CAD build for the part. Positions are in the model's coordinates, mm. A direction names the side the tool comes from. Coordinates: 2 decimals unless noted, no trailing zeros. Write each loop counter-clockwise with the first axis right and the second up, starting at its lowest first coordinate (ties: lowest second). Pieces come first, ordered by that corner, then holes. Notation, with made-up numbers: (60, 61) - (85, 61) arc R21 ccw to (85, 88) - close; hole circle Ø8 at (22.5, 62). An arc over 180 degrees is marked (long way). Answer in a Markdown table with one row per item. Add a question column.
Q1. Two-plate mould, pull along X, no slides. Class faces 5 (the flat face through (2, 6.35, 2)), 6 (the flat face through (47.997, 20, 2)): +X half, -X half, draft (parallel to the pull), parting line (faces both ways), or undercut.
Q2. Pin check, flat tips, straight feed: pin 1 (0.9 mm diameter, centred on y = 9, z = 2, fed in from -X) (3 decimals); pin 2 (1.6 mm diameter, centred on x = 11.5, z = 2, fed in from -Y) (3 decimals). Stop position of each tip, or through.
Q3. Band-saw the part on C-C (y = 5). State how many separate pieces and enclosed holes the cut face has, and give its area (3 significant figures).
Q4. Band-saw the part on B-B (x = 5). List the corners of the cut face in (y, z) (3 decimals), and give its area (3 significant figures).
Q5. 3-axis set-ups, long thin cutter, end or side, ignore diameter. For faces 1 (the flat face through (10, 25.4, 2)), 2 (the flat face through (2, 19.05, 2)), 3 (the flat face through (9.525, 9, 2)), 4 (the flat face through (15.875, 2, 2)): which of +Z, -Z, +X, -X, +Y, -Y reach the whole face in a straight line?
Q6. Drill centre lines: line 1 along Y through (x, z) = (4.5, 0.8) (3 decimals); line 2 along Y through (x, z) = (9, 1.95) (3 decimals). Where is each one in solid material? Low to high. Write a range as from..to.
Q7. Band-saw the part on A-A (x = 11). List the corners of the cut face in (y, z) (1 decimal).
```python
from build123d import *

# Parameters (mm, degrees)
BOSS_EXTRUDE2_DEPTH = 3.175


with BuildPart() as part:
    # Sketch1 → Boss-Extrude2 (new body)
    with BuildSketch(Plane.XY):
        Polygon((0, 6.35), (0, 0), (6.35, 0), (6.35, 3.175), (15.875, 3.175), (15.875, 0), (19.05, 0), (19.549044577, 11.43), (20.048089155, 0), (21.082, 0), (21.581044577, 11.43), (22.080089155, 0), (23.114, 0), (23.613044577, 11.43), (24.112089155, 0), (25.146, 0), (25.645044577, 11.43), (26.144089155, 0), (27.178, 0), (27.677044577, 11.43), (28.176089155, 0), (29.21, 0), (29.709044577, 11.43), (30.208089155, 0), (31.242, 0), (31.741044577, 11.43), (32.240089155, 0), (33.274, 0), (33.773044577, 11.43), (34.272089155, 0), (35.306, 0), (35.805044577, 11.43), (36.304089155, 0), (37.338, 0), (37.837044577, 11.43), (38.336089155, 0), (39.37, 0), (39.869044577, 11.43), (40.368089155, 0), (41.402, 0), (41.901044577, 11.43), (42.400089155, 0), (43.434, 0), (43.933044577, 11.43), (44.432089155, 0), (45.466, 0), (45.965044577, 11.43), (46.464089155, 0), (47.498, 0), (47.997044577, 11.43), (47.997044577, 0), (50.8, 0), (50.8, 25.4), (47.997044577, 25.4), (47.997044577, 13.97), (47.498, 25.4), (46.464089155, 25.4), (45.965044577, 13.97), (45.466, 25.4), (44.432089155, 25.4), (43.933044577, 13.97), (43.434, 25.4), (42.400089155, 25.4), (41.901044577, 13.97), (41.402, 25.4), (40.368089155, 25.4), (39.869044577, 13.97), (39.37, 25.4), (38.336089155, 25.4), (37.837044577, 13.97), (37.338, 25.4), (36.304089155, 25.4), (35.805044577, 13.97), (35.306, 25.4), (34.272089155, 25.4), (33.773044577, 13.97), (33.274, 25.4), (32.240089155, 25.4), (31.741044577, 13.97), (31.242, 25.4), (30.208089155, 25.4), (29.709044577, 13.97), (29.21, 25.4), (28.176089155, 25.4), (27.677044577, 13.97), (27.178, 25.4), (26.144089155, 25.4), (25.645044577, 13.97), (25.146, 25.4), (24.112089155, 25.4), (23.613044577, 13.97), (23.114, 25.4), (22.080089155, 25.4), (21.581044577, 13.97), (21.082, 25.4), (20.048089155, 25.4), (19.549044577, 13.97), (19.05, 25.4), (0, 25.4), (0, 19.05), (3.175, 19.05), (3.175, 14.605), (9.525, 14.605), (9.525, 17.4625), (12.7, 17.4625), (12.7, 14.605), (14.224, 14.605), (14.224, 10.795), (12.7, 10.795), (12.7, 7.9375), (9.525, 7.9375), (9.525, 10.795), (3.175, 10.795), (3.175, 6.35), align=None)
        Polygon((20.066, 12.7), (20.565044577, 24.13), (21.064089155, 12.7), (20.565044577, 1.27), align=None, mode=Mode.SUBTRACT)
        Polygon((22.098, 12.7), (22.597044577, 24.13), (23.096089155, 12.7), (22.597044577, 1.27), align=None, mode=Mode.SUBTRACT)
        Polygon((24.13, 12.7), (24.629044577, 24.13), (25.128089155, 12.7), (24.629044577, 1.27), align=None, mode=Mode.SUBTRACT)
        Polygon((26.162, 12.7), (26.661044577, 24.13), (27.160089155, 12.7), (26.661044577, 1.27), align=None, mode=Mode.SUBTRACT)
        Polygon((28.194, 12.7), (28.693044577, 24.13), (29.192089155, 12.7), (28.693044577, 1.27), align=None, mode=Mode.SUBTRACT)
        Polygon((30.226, 12.7), (30.725044577, 24.13), (31.224089155, 12.7), (30.725044577, 1.27), align=None, mode=Mode.SUBTRACT)
        Polygon((32.258, 12.7), (32.757044577, 24.13), (33.256089155, 12.7), (32.757044577, 1.27), align=None, mode=Mode.SUBTRACT)
        Polygon((34.29, 12.7), (34.789044577, 24.13), (35.288089155, 12.7), (34.789044577, 1.27), align=None, mode=Mode.SUBTRACT)
        Polygon((36.322, 12.7), (36.821044577, 24.13), (37.320089155, 12.7), (36.821044577, 1.27), align=None, mode=Mode.SUBTRACT)
        Polygon((38.354, 12.7), (38.853044577, 24.13), (39.352089155, 12.7), (38.853044577, 1.27), align=None, mode=Mode.SUBTRACT)
        Polygon((40.386, 12.7), (40.885044577, 24.13), (41.384089155, 12.7), (40.885044577, 1.27), align=None, mode=Mode.SUBTRACT)
        Polygon((42.418, 12.7), (42.917044577, 24.13), (43.416089155, 12.7), (42.917044577, 1.27), align=None, mode=Mode.SUBTRACT)
        Polygon((44.45, 12.7), (44.949044577, 24.13), (45.448089155, 12.7), (44.949044577, 1.27), align=None, mode=Mode.SUBTRACT)
        Polygon((46.482, 12.7), (46.981044577, 24.13), (47.480089155, 12.7), (46.981044577, 1.27), align=None, mode=Mode.SUBTRACT)
    extrude(amount=BOSS_EXTRUDE2_DEPTH)


solid = part.part
```
Checked values:
| question | item | result |
|---|---|---|
| 1 | face 5 | draft |
| 1 | face 6 | undercut |
| 2 | pin 1 | stops at x = 3.175 |
| 2 | pin 2 | stops at y = 3.175 |
| 3 | separate pieces | 30 |
| 3 | enclosed holes | 0 |
| 3 | area | 121 mm² |
| 4 | outline | (0, 0) - (10.795, 0) - (10.795, 3.175) - (0, 3.175) - close; (14.605, 0) - (25.4, 0) - (25.4, 3.175) - (14.605, 3.175) - close |
| 4 | area | 68.5 mm² |
| 5 | face 1 | +Z, -Z, +X, -X, +Y |
| 5 | face 2 | +Z, -Z, -X |
| 5 | face 3 | +Z, -Z |
| 5 | face 4 | +Z, -Z, -Y |
| 6 | line 1 | y = 0..10.795, 14.605..25.4 |
| 6 | line 2 | y = 3.175..10.795, 14.605..25.4 |
| 7 | outline | (3.2, 0) - (7.9, 0) - (7.9, 3.2) - (3.2, 3.2) - close; (17.5, 0) - (25.4, 0) - (25.4, 3.2) - (17.5, 3.2) - close |
